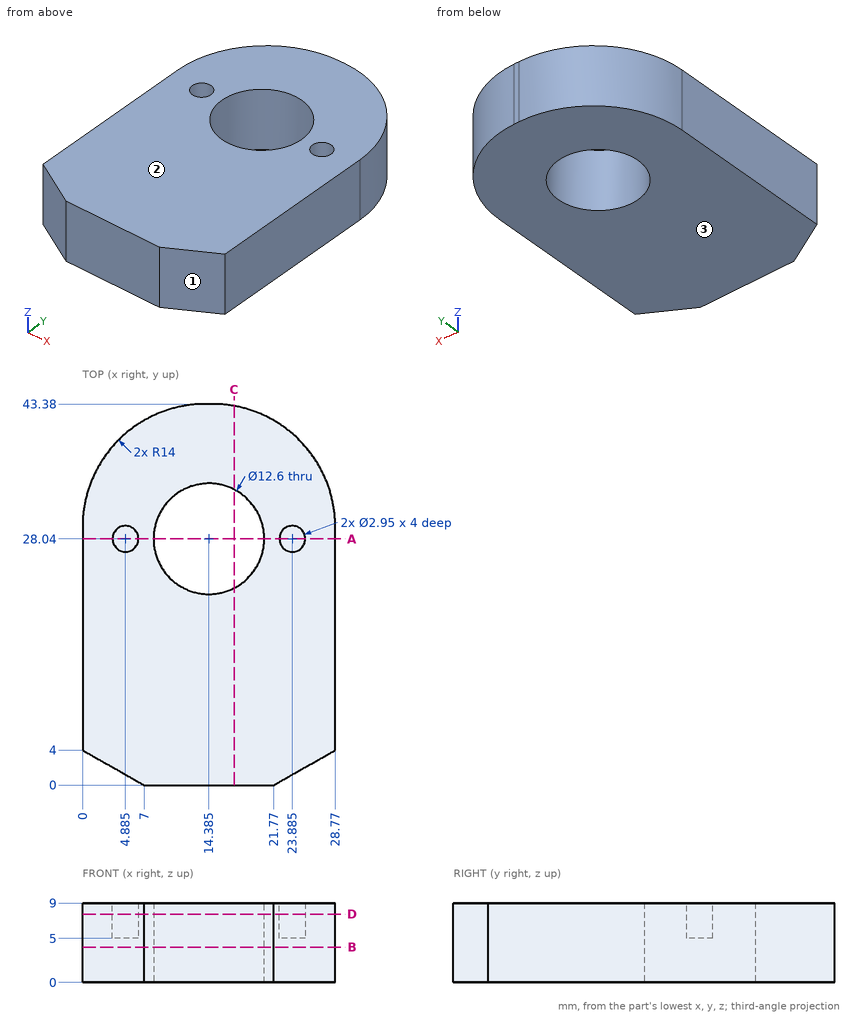
Can you work these out from the drawing? Everything is in mm from the part's minimum corner. Coordinates: 2 decimals unless noted, no trailing zeros. Order: outer loops, then holes, each group sorted by start corner. A loop starts at its lowest first (then second) coordinate and runs counter-clockwise, first axis right, second up. Notation, with made-up numbers: (71.5, -21.75) -> (116.5, -21.75) arc R19 cw to (116.5, -5.75) -> close; hole circle Ø3 at (79.5, 77). An arc over 180 degrees is marked (long way). Use one line per item in the form item = value.
Q1. Imagine slicing it at D-D, the plane z = 7.75. List the corners of the cut face in (x, y) for me (3 decimals), then the cut area to 3 significant figures.
From the geometry:
outline = (0, 4) -> (7, 0) -> (21.77, 0) -> (28.77, 4) -> (28.77, 29.38) arc R14 ccw to (14.77, 43.38) -> (14, 43.38) arc R14 ccw to (0, 29.38) -> close; hole circle Ø2.95 at (4.885, 28.04); hole circle Ø12.6 at (14.385, 28.04); hole circle Ø2.95 at (23.885, 28.04)
area = 998 mm²
Q2. Imagine slicing it at B-B, the plane z = 4. List the corners of the cut face in (x, y) for me (3 decimals).
From the geometry:
outline = (0, 4) -> (7, 0) -> (21.77, 0) -> (28.77, 4) -> (28.77, 29.38) arc R14 ccw to (14.77, 43.38) -> (14, 43.38) arc R14 ccw to (0, 29.38) -> close; hole circle Ø12.6 at (14.385, 28.04)
Q3. I need wall thicknesses on L1, parallel to Y at x = 19, z = 5; L2, parallel to Y at x = 17, z = 7.25; L3, parallel to X at y = 31, z = 3.5. Which ranges of each line are inside material? Lowest first, please.
From the geometry:
L1 = 0 to 23.75, 32.33 to 42.73
L2 = 0 to 22.31, 33.77 to 43.2
L3 = 0.09 to 8.82, 19.95 to 28.68
Q4. We'd pull the mould along Z, two halves only. Please class the marked faces 1, 2 and 3: released by +Z, released by -Z, zero draft, split by the parting line, or undercut.
From the geometry:
face_1 = zero draft
face_2 = released by +Z
face_3 = released by -Z
Q5. Will these pins go through, and if not, where does the flat tip stop? P1, Ø11.5, axis at x = 14.385, y = 28.04, coming from the -Z side; P2, Ø2, axis at y = 39, z = 6.5, coming from the +X side; P3, Ø1, axis at x = 9, z = 4.5, coming from the +Y side; P4, Ø1.8, axis at x = 4.885, y = 28.04, coming from the +Z side.
From the geometry:
P1 = through
P2 = 25.8
P3 = 42.64
P4 = 5
Q6. Imagine slicing it at A-A, the plane y = 28.04. List the corners of the cut face in (x, z) for me (3 decimals).
From the geometry:
outline = (0, 0) -> (8.085, 0) -> (8.085, 9) -> (6.36, 9) -> (6.36, 5) -> (3.41, 5) -> (3.41, 9) -> (0, 9) -> close; (20.685, 0) -> (28.77, 0) -> (28.77, 9) -> (25.36, 9) -> (25.36, 5) -> (22.41, 5) -> (22.41, 9) -> (20.685, 9) -> close
Q7. Imagine slicing it at C-C, the plane x = 17.25. List the corners of the cut face in (y, z) for me, then the cut area to 3 significant figures.
From the geometry:
outline = (0, 0) -> (22.43, 0) -> (22.43, 9) -> (0, 9) -> close; (33.65, 0) -> (43.16, 0) -> (43.16, 9) -> (33.65, 9) -> close
area = 287 mm²
